```python
from build123d import *

# Parameters (mm, degrees)
F0_R          = 51.562
F0_R_2        = 47.5
F1_DEPTH      = 196.85
F3_DEPTH      = 61
F3_DEPTH_BACK = 74
F4_W          = 38.1
F4_H          = 101.6
F5_DEPTH      = 61
F8_DEPTH      = 103.1
F10_DEPTH     = 222
F12_R         = 35.605551274
F13_DEPTH     = 6.3
F14_R         = 47.7557531621
F15_DEPTH     = 4


with BuildPart() as f1:
    # F0 (on Top) → F1 (new body)
    with BuildSketch(Plane.XY):
        Circle(F0_R)
        Circle(F0_R_2, mode=Mode.SUBTRACT)
    extrude(amount=F1_DEPTH)

    # F2 (on Front) → F3 (cut, two sides)
    with BuildSketch(Plane.XZ) as f3_sk:
        Polygon((-53.9132580161, 197.3211467266), (-51.5358708799, 168.91), (53.5786189139, 197.3211467266), align=None)
    extrude(amount=F3_DEPTH, mode=Mode.SUBTRACT)
    extrude(f3_sk.sketch, amount=-F3_DEPTH_BACK, mode=Mode.SUBTRACT)

    # F4 (on Right) → F5 (cut)
    with BuildSketch(Plane.YZ):
        with Locations((0.9657477468, 50.8)):
            Rectangle(F4_W, F4_H)
    extrude(amount=-F5_DEPTH, mode=Mode.SUBTRACT)

    # F7 (on offset) → F8 (join)
    with BuildSketch(Plane.XZ.offset(51.59)):
        Polygon((-51.558252424, 169.7267442942), (-51.558252424, 168.8925474882), (51.5620075166, 196.7761367559), (51.5620075166, 197.6103335619), align=None)
    extrude(amount=-F8_DEPTH)

    # F9 (on Top) → F10 (cut)
    with BuildSketch(Plane.XY):
        Polygon((-55.258795619, 55.1219135523), (-55.258795619, 0), (-55.258795619, -56.1094321311), (54.045163095, -56.1094321311), (54.045163095, 51.9001446664), align=None)
        with BuildLine():
            ThreePointArc((-51.776278764, 0), (-36.3661223593, 36.403048351), (0, 51.9001446664))
            ThreePointArc((0, 51.9001446664), (36.452456, 36.4891781459), (51.7762713134, 0))
            ThreePointArc((51.7762713134, 0), (36.3947916683, -36.3580565829), (0, -51.6524128616))
            ThreePointArc((0, -51.6524128616), (-36.4887208542, -36.4522087985), (-51.776278764, 0))
        make_face(mode=Mode.SUBTRACT)
    extrude(amount=F10_DEPTH, mode=Mode.SUBTRACT)

    # F12 (on offset) → F13 (cut)
    with BuildSketch(Plane(origin=(-46.3581408372, 0, 171.4436218234), x_dir=(0.9653321478, 0, 0.261024605), z_dir=(-0.261024605, 0, 0.9653321478))):
        with Locations((48.5923029482, 0)):
            Circle(F12_R)
    extrude(amount=-F13_DEPTH, mode=Mode.SUBTRACT)

    # F14 (on Top) → F15 (join)
    with BuildSketch(Plane.XY):
        Circle(F14_R)
    extrude(amount=-F15_DEPTH)


solid = f1.part
```
Verification items for the finished model (mm, model axes). A direction names the side the tool comes from. Give positions to 0.01 mm unless a question says otherwise; leave off trailing zeros. Order: outer loops, then holes, each group sorted by start corner. A loop starts at its lowest first (then second) coordinate and runs counter-clockwise, first axis right, second up. Notation, with made-up numbers: (1, 13.5) -> (31, 13.5) arc R19 cw to (31, 49.5) -> close; hole circle Ø8 at (85, 13.5). An arc over 180 degrees is marked (long way). Use a Markdown table: item, result.
1) Section check D-D, the plane z = 113. Record the boundary of the cut face in (x, y), then the cut area to 3 significant figures.
Results:
| item | result |
|---|---|
| outline | (-49.16, 15.56) arc R51.56 ccw to (8.8, -50.81) arc R52.38 ccw to (48.25, -18.18) arc R51.56 ccw to (-21.96, 46.65) arc R52.79 ccw to start; hole circle Ø95 at (0, 0) |
| area | 1,260 mm² |
2) Mould release check, pull along X, two halves, no side actions. Record for faces 3 (the cylindrical face through (45.307, 14.268, 96.469)), 4 (the flat face through (-45, 20.016, 50)), 5 (the flat face through (-33.65, 10.69, 174.57)): pulls with the +X half, pulls with the -X half, needs draft (parallel to the pull), parting line crosses it, or undercut.
Results:
| item | result |
|---|---|
| face 3 | undercut |
| face 4 | needs draft |
| face 5 | pulls with the -X half |
3) Tool access check on faces 1 (the cylindrical face through (45.55, 14.34, -1.97)), 2 (the flat face through (-32.332, 9.891, 174.091)). Record the directions out of +Z, -Z, +X, -X, +Y, -Y that give a thin tool (end or side, any length) a straight path to the whole face; none if there is none.
Results:
| item | result |
|---|---|
| face 1 | -Z |
| face 2 | none |
4) Material ranges on probe 1 along X at (y, z) = (0, 123); probe 2 along Z at (x, y) = (-12, -20), recorded low to high.
Results:
| item | result |
|---|---|
| probe 1 | -51.56 to -47.5, 47.5 to 51.56 |
| probe 2 | -4 to 0 |
5) Depth check by flat-ended pin: pin 1 Ø5 at (y, z) = (-24.5, 127.5) entering from -X; pin 2 Ø4 at (x, z) = (40, 163) entering from -Y; pin 3 Ø6 at (x, z) = (-18.5, 116.5) entering from +Y. Enter the tip coordinate at first touch or a pass-through.
Results:
| item | result |
|---|---|
| pin 1 | x = -46.63 |
| pin 2 | y = -34.68 |
| pin 3 | y = 49.18 |
